Geometry check sheet. Reference: drawing and pictorial views, mm from the part's lowest x, y, z. A direction names the side the tool comes from. Round coordinates to 2 decimals unless told otherwise and drop trailing zeros. Write each loop counter-clockwise with the first axis right and the second up, starting at its lowest first coordinate (ties: lowest second). Pieces come first, ordered by that corner, then holes.
Item 1: Set-up check for the marked faces 5 and 6: record each of +Z, -Z, +X, -X, +Y, -Y from which the full face is reachable in a straight line by a thin tool's end or side.
Item 2: Section check D-D, the plane y = 5.75. Record the cut outline in (x, z) (3 decimals), plus the area to 3 significant figures.
Item 3: Material ranges on line 1 along Y through (x, z) = (6.35, 11.05) (3 decimals); line 2 along Z through (x, y) = (9.25, 4.5) (3 decimals); line 3 along Y through (x, z) = (1.5, 2.25) (3 decimals), recorded low to high.
Item 4: Section check A-A, the plane y = 20.32. Record the cut outline in (x, z) (3 decimals), plus the area to 3 significant figures.
Item 5: Section check B-B, the plane x = 7.5. Record the cut outline in (y, z) (3 decimals), plus the area to 3 significant figures.
Item 6: Release check for a two-part mould opening along Y. For the marked faces 1, 2, 3 and 4 record: pulls with the +Y half, pulls with the -Y half, needs draft (parallel to the pull), parting line crosses it, or undercut.
Item 7: Section check C-C, the plane x = 3.75. Record the cut outline in (y, z) (3 decimals), plus the area to 3 significant figures.
Item 8: Depth check by flat-ended pin: pin 1 (4 mm diameter, centred on x = 6.5, y = 13, fed in from -Z) (3 decimals); pin 2 (5 mm diameter, centred on x = 6.35, y = 20.32, fed in from -Z); pin 3 (5 mm diameter, centred on x = 8, z = 4, fed in from +Y) (3 decimals). Enter the tip coordinate at first touch or a pass-through.
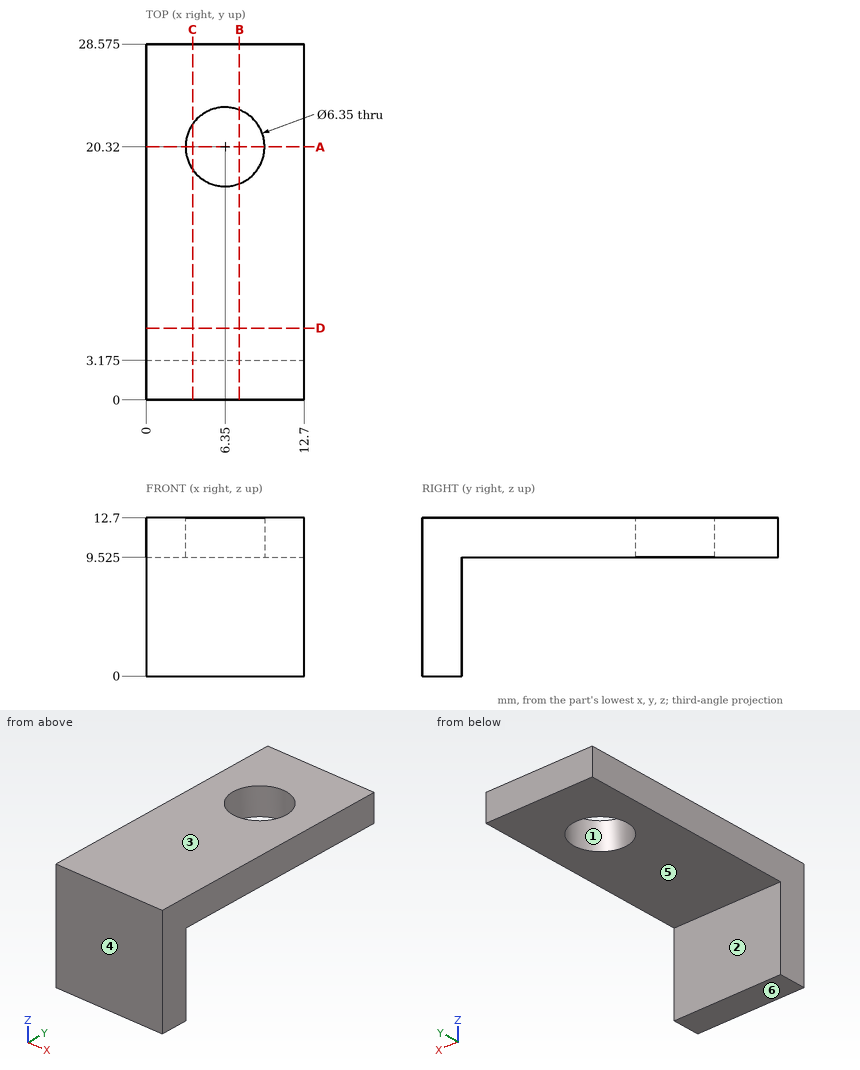
Values found:
1. face 5: -Z, +X, -X, +Y
1. face 6: -Z, +X, -X, +Y, -Y
2. outline: (0, 9.525) - (12.7, 9.525) - (12.7, 12.7) - (0, 12.7) - close
2. area: 40.3 mm2
3. line 1: y = 0 to 17.145, 23.495 to 28.575
3. line 2: z = 9.525 to 12.7
3. line 3: y = 0 to 3.175
4. outline: (0, 9.525) - (3.175, 9.525) - (3.175, 12.7) - (0, 12.7) - close; (9.525, 9.525) - (12.7, 9.525) - (12.7, 12.7) - (9.525, 12.7) - close
4. area: 20.2 mm2
5. outline: (0, 0) - (3.175, 0) - (3.175, 9.525) - (17.361, 9.525) - (17.361, 12.7) - (0, 12.7) - close; (23.279, 9.525) - (28.575, 9.525) - (28.575, 12.7) - (23.279, 12.7) - close
5. area: 102 mm2
6. face 1: undercut
6. face 2: pulls with the +Y half
6. face 3: needs draft
6. face 4: pulls with the -Y half
7. outline: (0, 0) - (3.175, 0) - (3.175, 9.525) - (18.498, 9.525) - (18.498, 12.7) - (0, 12.7) - close; (22.142, 9.525) - (28.575, 9.525) - (28.575, 12.7) - (22.142, 12.7) - close
7. area: 109 mm2
8. pin 1: stops at z = 9.525
8. pin 2: passes through
8. pin 3: stops at y = 3.175
